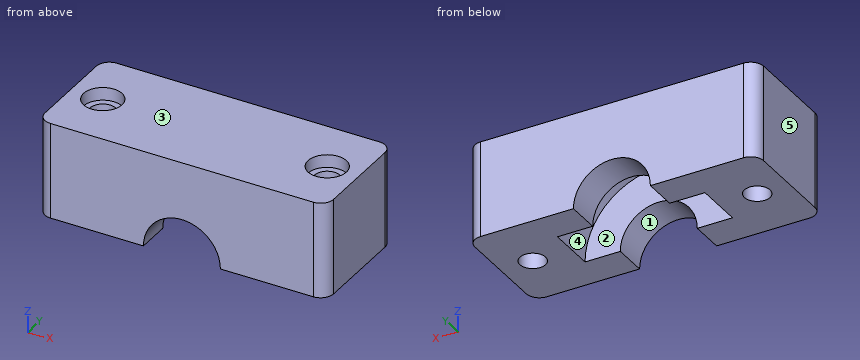
Autodesk Inventor part; units mm, degrees
ref_plane "YZ Plane" through (0, 0, 0) normal (1, 0, 0) x (0, 1, 0)
ref_plane "XZ Plane" through (0, 0, 0) normal (0, 1, 0) x (-1, 0, 0)
ref_plane "XY Plane" through (0, 0, 0) normal (0, 0, 1) x (1, 0, 0)
sketch "Sketch1" plane through (0, 0, 0) normal (0, 0, 1) x (1, 0, 0)
  point P0 (0, 0)
sketch "Sketch2" plane through (0, 0, 0) normal (0, 0, 1) x (1, 0, 0)
  line L0 (-22.5, 9) -> (22.5, 9)
  line L1 (22.5, 9) -> (22.5, -9)
  line L2 (22.5, -9) -> (-22.5, -9)
  line L3 (-22.5, -9) -> (-22.5, 9)
  line L4 (-22.5, 9) -> (22.5, -9) construction
  line L5 (22.5, 9) -> (-22.5, -9) construction
  point P0 (0, 0)
  dimension "d0" = 45
  dimension "d1" = 18
extrude "Extrusion1" add sketch "Sketch2" along normal blind 15
ref_plane "Work Plane1" through (-22.5, 0, 0) normal (0, 1, 0) x (1, 0, 0)
sketch "Sketch3" plane through (-22.5, 0, 0) normal (0, 1, 0) x (1, 0, 0)
  circle A0 centre (22.5, 0) radius 11.5
  dimension "d4" = 23
extrude "Extrusion2" cut sketch "Sketch3" along normal mid plane 7.5
sketch "Sketch4" plane through (-22.5, 0, 0) normal (0, 1, 0) x (1, 0, 0)
  circle A0 centre (22.5, 0) radius 6
  dimension "d7" = 12
extrude "Extrusion3" cut sketch "Sketch4" along normal mid plane 32.75
sketch "Sketch5" plane through (0, 0, 15) normal (0, 0, 1) x (1, 0, 0)
  line L0 (-22.5, 9) -> (-22.5, -9)
  line L1 (-22.5, -9) -> (22.5, -9)
  point P0 (0, 0)
  point P1 (-17.5, 0)
  dimension "d10" = 5
  dimension "d11" = 9
hole "Hole1" at (-17.5, 0, 15) direction (0, 0, -1) diameter 4 end through all counterbore diameter 6 counterbore depth 2
sketch "Sketch6" plane through (0, 0, 15) normal (0, 0, 1) x (1, 0, 0)
  line L0 (-22.5, -9) -> (22.5, -9)
  line L1 (22.5, -9) -> (22.5, 9)
  point P0 (0, 0)
  point P1 (17.5, 0)
  dimension "d19" = 9
  dimension "d20" = 5
hole "Hole2" at (17.5, 0, 15) direction (0, 0, -1) diameter 4 end through all counterbore diameter 6 counterbore depth 2
fillet "Fillet1" radius 2 4 edges at (-22.5, -9, 7.5) (22.5, -9, 7.5) (-22.5, 9, 7.5) (22.5, 9, 7.5)
properties part number "bearing_holder_v2"
CAD build for the part. Positions are in the model's coordinates, mm. Face numbers are marked on the shaded views. A direction names the side the tool comes from. Give positions to 0.01 mm unless a question says otherwise; leave off trailing zeros. Write each loop counter-clockwise with the first axis right and the second up, starting at its lowest first coordinate (ties: lowest second). Pieces come first, ordered by that corner, then holes. Notation, with made-up numbers: M 79.25,11.25 L 136.25,11.25 A13 cw 136.25,27.25 Z; hole C -14.75,71 d2. An arc over 180 degrees is marked long. Put each result on its own line as item: value. Start each with the question number.
(1) Band-saw the part on A-A, the plane x = -17.5. Write the cut outline in (y, z).
(2) Which spindle directions (+Z, -Z, +X, -X, +Y, -Y) get a long thin tool onto all of the face, cutting with end or side? Do the marked faces 1 and 2. Say none if no direction does.
(3) Band-saw the part on B-B, the plane y = 0. Write the cut outline in (x, z), and give its area (3 significant figures).
(4) Band-saw the part on C-C, the plane x = 0. Write the cut outline in (y, z).
(5) Mould opens along X. For the marked faces 3, 4 and 5 say: +X half, -X half, draft (parallel to the pull), parting line (faces both ways), or undercut.
(6) Probe L1, parallel to X at y = 0, z = 14; L2, parallel to X at y = 0, z = 5.75; L3, parallel to Y at x = 17.5, z = 14.4. List the from-to ranges inside material, lowest first.
(7) Band-saw the part on D-D, the plane z = 7.25. Write the cut outline in (x, y).
Response values:
1. outline: M -9,0 L -2,0 L -2,13 L -3,13 L -3,15 L -9,15 Z; M 2,0 L 9,0 L 9,15 L 3,15 L 3,13 L 2,13 Z
2. face 1: -Z, +Y, -Y
2. face 2: -Z
3. outline: M -22.5,0 L -19.5,0 L -19.5,13 L -20.5,13 L -20.5,15 L -22.5,15 Z; M -15.5,0 L -11.5,0 A11.5 cw 11.5,0 L 15.5,0 L 15.5,13 L 14.5,13 L 14.5,15 L -14.5,15 L -14.5,13 L -15.5,13 Z; M 19.5,0 L 22.5,0 L 22.5,15 L 20.5,15 L 20.5,13 L 19.5,13 Z
3. area: 339 mm2
4. outline: M -9,6 L -3.75,6 L -3.75,11.5 L 3.75,11.5 L 3.75,6 L 9,6 L 9,15 L -9,15 Z
5. face 3: draft
5. face 4: undercut
5. face 5: -X half
6. L1: x = -22.5 to -20.5, -14.5 to 14.5, 20.5 to 22.5
6. L2: x = -22.5 to -19.5, -15.5 to -9.96, 9.96 to 15.5, 19.5 to 22.5
6. L3: y = -9 to -3, 3 to 9
7. outline: M -22.5,-7 A2 ccw -20.5,-9 L 20.5,-9 A2 ccw 22.5,-7 L 22.5,7 A2 ccw 20.5,9 L -20.5,9 A2 ccw -22.5,7 Z; hole C -17.5,0 d4; hole M -8.93,-3.75 L 8.93,-3.75 L 8.93,3.75 L -8.93,3.75 Z; hole C 17.5,0 d4
